```python
from build123d import *

# Parameters (mm, degrees)
SKETCH1_R           = 2.44543137
BOSS_EXTRUDE1_DEPTH = 5
SKETCH2_W           = 3.567027941
SKETCH2_H           = 2.066611426
BOSS_EXTRUDE2_DEPTH = 0.4
SWEEP2_PROFILE_R    = 0.5


with BuildPart() as part:
    # Sketch1 → Boss-Extrude1 (new body)
    with BuildSketch(Plane(origin=(0, 0, 0), x_dir=(1, 0, 0), z_dir=(0, 1, 0))):
        with BuildLine():
            Line((-4.846115072, 4), (4.846115072, 4))
            ThreePointArc((4.846115072, 4), (8.846115072, 0), (4.846115072, -4))
            Line((4.846115072, -4), (-4.846115072, -4))
            ThreePointArc((-4.846115072, -4), (-8.846115072, 0), (-4.846115072, 4))
        make_face()
        Circle(SKETCH1_R, mode=Mode.SUBTRACT)
    extrude(amount=BOSS_EXTRUDE1_DEPTH)

    # Sketch2 → Boss-Extrude2 (add)
    with BuildSketch(Plane(origin=(0, 5, 0), x_dir=(1, 0, 0), z_dir=(0, 1, 0))):
        with Locations((-5.407161402, 0)):
            Rectangle(SKETCH2_W, SKETCH2_H)
    boss_extrude2 = extrude(amount=BOSS_EXTRUDE2_DEPTH)

    # Sweep2: sweep along a path in Sketch3
    with BuildLine(Plane.XY) as sweep2_path:
        Line((-6.34863908, 5.4), (-6.34863908, 6.437017348))
        ThreePointArc((-6.34863908, 6.437017348), (-5.367322582, 7.418333845), (-4.386006084, 6.437017348))
    # Sweep2 profile (on start of the path) → Sweep2 (sweep)
    with BuildSketch(Plane(origin=(-6.34863908, 5.4, 0), x_dir=(0, 0, 1), z_dir=(0, 1, 0))):
        Circle(SWEEP2_PROFILE_R)
    sweep2 = sweep(path=sweep2_path.line)

    # Mirror1: Boss-Extrude2, Sweep2 across plane
    add(boss_extrude2.mirror(Plane(origin=(0, 0, 0), x_dir=(0, 0, 1), z_dir=(1, 0, 0))))
    add(sweep2.mirror(Plane(origin=(0, 0, 0), x_dir=(0, 0, 1), z_dir=(1, 0, 0))))


solid = part.part
```
Work out the finished part from the listing and answer in its coordinate system (mm). A direction names the side the tool comes from. Give positions to 0.01 mm unless a question says otherwise; leave off trailing zeros. Loops run counter-clockwise (first coordinate to the right, second up) from the corner with the lowest first, then second, coordinate; pieces in that order, holes last. Notation, with made-up numbers: (67, 24.5) -> (111, 24.5) arc R27 ccw to (111, 48.5) -> close; hole circle Ø4 at (78.25, -11.5). An arc over 180 degrees is marked (long way). One line per question, with ' | ' between items. Start each with the question number.
1) Section B-B, the plane x = 0 is taken. Determine the outline of the cut face in (y, z), then the cut area to 3 significant figures.
2) Determine the mould class of faces 1 (the face through (-6.792, 5.926, 0.231)), 2 (the face through (2.333, 2.465, -0.735)), 3 (the face through (-8.845, 2.465, 0.088)), 4 (the face through (0, 2, 4)) for opening direction X: +X half, -X half, draft (parallel to the pull), parting line (faces both ways), or undercut.
3) Section A-A, the plane z = 0 is taken. Determine the outline of the cut face in (x, y).
4) For faces 5 (the face through (4.4, 6.437, 0)), 6 (the face through (-2, 0, -2)), 7 (the face through (6.792, 5.926, 0.231)), determine the directions among +Z, -Z, +X, -X, +Y, -Y from which every point of the face is accessible in a straight line to the end or side of a thin tool.
5) Section D-D, the plane z = -1.25 is taken. Determine the outline of the cut face in (x, y), then the cut area to 3 significant figures.
6) Straight lines are drawn through the part: L1, parallel to Z at x = 0, y = 1.9; L2, parallel to X at y = 2.75, z = 0; L3, parallel to Y at x = 4.5, z = 3.25. For each, find the intervals that lie inside material, in ascending order.
7) Section C-C, the plane y = 3.75 is taken. Determine the outline of the cut face in (x, z).
8) Each of these flat-tipped pins is pushed along its axis until it touches: pin 1 (1 mm diameter, centred on y = 1, z = 1.5, fed in from -X); pin 2 (1 mm diameter, centred on x = -6.5, z = -1.5, fed in from +Y); pin 3 (1 mm diameter, centred on y = 3, z = 2, fed in from +X). Where does it stop, or does it pass through?
Resolved:
1) outline: (0, -4) -> (5, -4) -> (5, -2.45) -> (0, -2.45) -> close; (0, 2.45) -> (5, 2.45) -> (5, 4) -> (0, 4) -> close | area: 15.5 mm2
2) face 1: undercut | face 2: undercut | face 3: -X half | face 4: draft
3) outline: (-8.85, 0) -> (-2.45, 0) -> (-2.45, 5) -> (-3.62, 5) -> (-3.62, 5.4) -> (-5.85, 5.4) -> (-5.85, 6.44) arc R0.48 cw to (-4.89, 6.44) -> (-3.89, 6.44) arc R1.48 ccw to (-6.85, 6.44) -> (-6.85, 5.4) -> (-7.19, 5.4) -> (-7.19, 5) -> (-8.85, 5) -> close; (2.45, 0) -> (8.85, 0) -> (8.85, 5) -> (7.19, 5) -> (7.19, 5.4) -> (6.85, 5.4) -> (6.85, 6.44) arc R1.48 ccw to (3.89, 6.44) -> (4.89, 6.44) arc R0.48 cw to (5.85, 6.44) -> (5.85, 5.4) -> (3.62, 5.4) -> (3.62, 5) -> (2.45, 5) -> close
4) face 5: +Z, -Z | face 6: +Z, -Z, +X, -X, -Y | face 7: none
5) outline: (-8.65, 0) -> (-2.1, 0) -> (-2.1, 5) -> (-8.65, 5) -> close; (2.1, 0) -> (8.65, 0) -> (8.65, 5) -> (2.1, 5) -> close | area: 65.4 mm2
6) L1: -4 to -2.45, 2.45 to 4 | L2: -8.85 to -2.45, 2.45 to 8.85 | L3: 0 to 5
7) outline: (-4.85, -4) -> (4.85, -4) arc R4 ccw to (4.85, 4) -> (-4.85, 4) arc R4 ccw to start; hole circle Ø4.89 at (0, 0)
8) pin 1: x = -8.72 | pin 2: y = 5.4 | pin 3: x = 8.55
